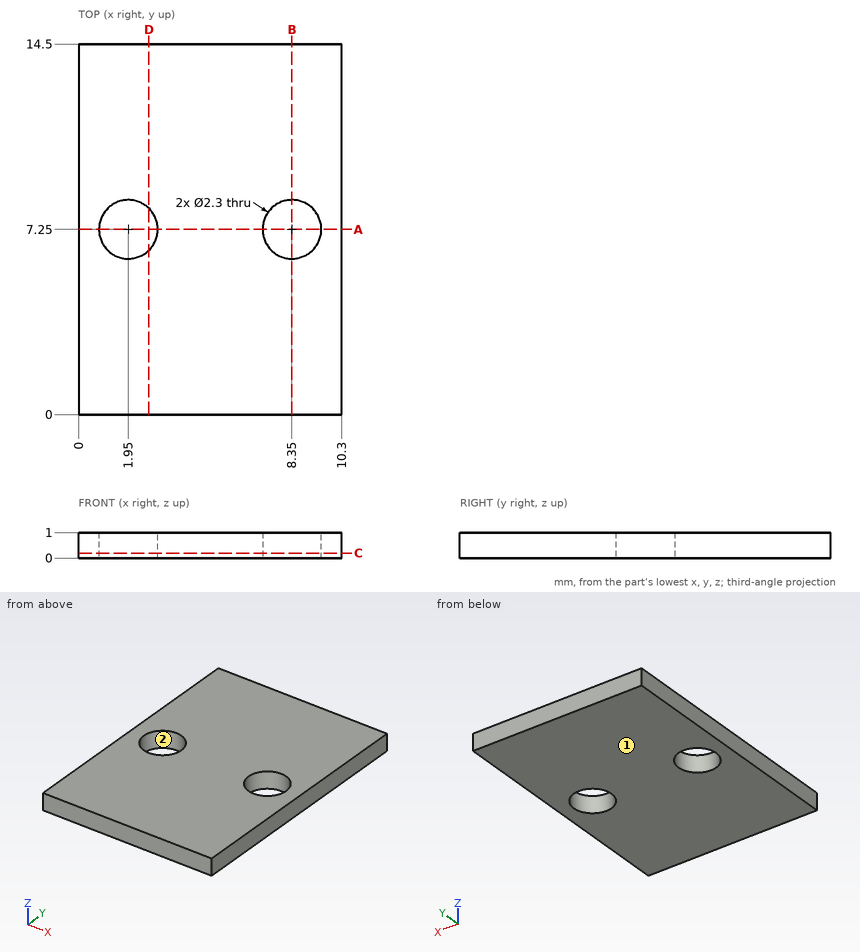
The figure shows three views and two pictorial views of one solid part (mm, origin at its lowest corner). Answer the questions. Round coordinates to 2 decimals unless told otherwise and drop trailing zeros. Write each loop counter-clockwise with the first axis right and the second up, starting at its lowest first coordinate (ties: lowest second). Pieces come first, ordered by that corner, then holes. Notation, with made-up numbers: (-10, -33.5) -> (24, -33.5) arc R22 ccw to (24, -24.5) -> close; hole circle Ø4 at (53.5, 61.5). An arc over 180 degrees is marked (long way). Answer as a JSON object with one key per item and string values. Group by question number.
Q1. Section C-C (z = 0.2) is taken. Write down the section's boundary in (x, y).
Q2. Section D-D (x = 2.75) is taken. Write down the section's boundary in (y, z).
Q3. Section B-B (x = 8.35) is taken. Write down the section's boundary in (y, z).
Q4. Straight lines are drawn through the part: line 1 along Y through (x, z) = (8.35, 0.3); line 2 along X through (y, z) = (6.25, 0.85); line 3 along Y through (x, z) = (7.5, 0.15). For each, find the intervals that lie inside material, in ascending order.
Q5. Section A-A (y = 7.25) is taken. Write down the section's boundary in (x, z), plus the area to 3 significant figures.
Q6. This flat-tipped pin is pushed along its axis until it touches: pin 1 Ø1.8 at (x, y) = (1.95, 7.25) entering from -Z. Where does it stop, or does it pass through?
Q7. Determine the mould class of the marked faces 1 and 2 for opening direction Y: pulls with the +Y half, pulls with the -Y half, needs draft (parallel to the pull), parting line crosses it, or undercut.
Check values:
{
 "1": {"outline": "(0, 0) -> (10.3, 0) -> (10.3, 14.5) -> (0, 14.5) -> close; hole circle Ø2.3 at (1.95, 7.25); hole circle Ø2.3 at (8.35, 7.25)"},
 "2": {"outline": "(0, 0) -> (6.42, 0) -> (6.42, 1) -> (0, 1) -> close; (8.08, 0) -> (14.5, 0) -> (14.5, 1) -> (8.08, 1) -> close"},
 "3": {"outline": "(0, 0) -> (6.1, 0) -> (6.1, 1) -> (0, 1) -> close; (8.4, 0) -> (14.5, 0) -> (14.5, 1) -> (8.4, 1) -> close"},
 "4": {"line 1": "0 to 6.1, 8.4 to 14.5", "line 2": "0 to 1.38, 2.52 to 7.78, 8.92 to 10.3", "line 3": "0 to 6.48, 8.02 to 14.5"},
 "5": {"outline": "(0, 0) -> (0.8, 0) -> (0.8, 1) -> (0, 1) -> close; (3.1, 0) -> (7.2, 0) -> (7.2, 1) -> (3.1, 1) -> close; (9.5, 0) -> (10.3, 0) -> (10.3, 1) -> (9.5, 1) -> close", "area": "5.70 mm^2"},
 "6": {"pin 1": "through"},
 "7": {"face 1": "needs draft", "face 2": "undercut"}
}
